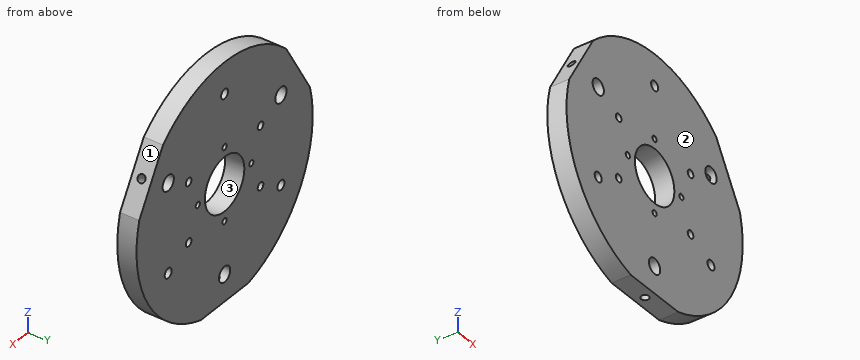
from build123d import *

# Parameters (mm, degrees)
SKETCH1_R           = 62.5
SKETCH1_R_2         = 4
BOSS_EXTRUDE1_DEPTH = 10
SKETCH2_W           = 43.972180284
SKETCH2_H           = 8.711954994
CUT_EXTRUDE1_DEPTH  = 10
SKETCH3_R           = 2
CUT_EXTRUDE2_DEPTH  = 12
SKETCH4_R           = 2
CUT_EXTRUDE3_DEPTH  = 12
SKETCH5_R           = 2
CUT_EXTRUDE4_DEPTH  = 12
SKETCH6_R           = 14
CUT_EXTRUDE5_DEPTH  = 12
SKETCH7_R           = 1.5
CUT_EXTRUDE6_DEPTH  = 10
SKETCH8_R           = 2
CUT_EXTRUDE7_DEPTH  = 10
SKETCH9_R           = 2.5
CUT_EXTRUDE8_DEPTH  = 10


with BuildPart() as part:
    # Sketch1 → Boss-Extrude1 (new body)
    with BuildSketch(Plane(origin=(0, 0, 0), x_dir=(1, 0, 0), z_dir=(0, 1, 0))):
        with Locations(Location((0, 0, 0), (0, 0, 270))):
            Circle(SKETCH1_R)
        with Locations(Location((0, 46.188021535, 0), (0, 0, 270))):
            Circle(SKETCH1_R_2, mode=Mode.SUBTRACT)
        with Locations(Location((40, -23.094010768, 0), (0, 0, 270))):
            Circle(SKETCH1_R_2, mode=Mode.SUBTRACT)
        with Locations(Location((-40, -23.094010768, 0), (0, 0, 270))):
            Circle(SKETCH1_R_2, mode=Mode.SUBTRACT)
    extrude(amount=BOSS_EXTRUDE1_DEPTH)

    # Sketch2 → Cut-Extrude1 (cut)
    with BuildSketch(Plane(origin=(0, 10, 0), x_dir=(1, 0, 0), z_dir=(0, 1, 0))):
        Polygon((-39.581845605, -51.818275424), (-64.713070734, -8.289716646), (-77.687460418, -15.780484023), (-52.55623529, -59.309042801), align=None)
        Polygon((40.609652539, -50.038061596), (63.321086643, -10.700703814), (75.641288558, -17.813775707), (52.929854454, -57.151133488), align=None)
        with Locations((0.471086747, 64.543999032)):
            Rectangle(SKETCH2_W, SKETCH2_H)
    extrude(amount=-CUT_EXTRUDE1_DEPTH, mode=Mode.SUBTRACT)

    # Sketch3 → Cut-Extrude2 (cut)
    with BuildSketch(Plane(origin=(52.124355653, 0, 30.094010768), x_dir=(0.49999999999999983, 0, -0.8660254037844387), z_dir=(0.8660254037844387, 0, 0.49999999999999983))):
        with Locations((0.001973272, 5)):
            Circle(SKETCH3_R)
    extrude(amount=-CUT_EXTRUDE2_DEPTH, mode=Mode.SUBTRACT)

    # Sketch4 → Cut-Extrude3 (cut)
    with BuildSketch(Plane(origin=(-52.124355653, 0, 30.094010768), x_dir=(0.5000000000000002, 0, 0.8660254037844386), z_dir=(-0.8660254037844385, 0, 0.5000000000000001))):
        with Locations((-0.001973272, 5)):
            Circle(SKETCH4_R)
    extrude(amount=-CUT_EXTRUDE3_DEPTH, mode=Mode.SUBTRACT)

    # Sketch5 → Cut-Extrude4 (cut)
    with BuildSketch(Plane(origin=(0, 0, -60.188021535), x_dir=(-1, 0, 0), z_dir=(0, 0, -1))):
        with Locations((-0.001973272, 5)):
            Circle(SKETCH5_R)
    extrude(amount=-CUT_EXTRUDE4_DEPTH, mode=Mode.SUBTRACT)

    # Sketch6 → Cut-Extrude5 (cut)
    with BuildSketch(Plane(origin=(0, 10, 0), x_dir=(1, 0, 0), z_dir=(0, 1, 0))):
        with Locations(Location((0, 0, 0), (0, 0, 270))):
            Circle(SKETCH6_R)
    extrude(amount=-CUT_EXTRUDE5_DEPTH, mode=Mode.SUBTRACT)

    # Sketch7 → Cut-Extrude6 (cut)
    with BuildSketch(Plane(origin=(0, 10, 0), x_dir=(1, 0, 0), z_dir=(0, 1, 0))):
        with Locations(Location((0, 19, 0), (0, 0, 270))):
            Circle(SKETCH7_R)
        with Locations(Location((19, 0, 0), (0, 0, 270))):
            Circle(SKETCH7_R)
        with Locations(Location((0, -19, 0), (0, 0, 270))):
            Circle(SKETCH7_R)
        with Locations(Location((-19, 0, 0), (0, 0, 270))):
            Circle(SKETCH7_R)
    extrude(amount=-CUT_EXTRUDE6_DEPTH, mode=Mode.SUBTRACT)

    # Sketch8 → Cut-Extrude7 (cut)
    with BuildSketch(Plane(origin=(0, 10, 0), x_dir=(1, 0, 0), z_dir=(0, 1, 0))):
        with Locations(Location((-25.5, 15.5, 0), (0, 0, 270))):
            Circle(SKETCH8_R)
        with Locations(Location((25.5, 15.5, 0), (0, 0, 270))):
            Circle(SKETCH8_R)
        with Locations(Location((25.5, -15.5, 0), (0, 0, 270))):
            Circle(SKETCH8_R)
        with Locations(Location((-25.5, -15.5, 0), (0, 0, 270))):
            Circle(SKETCH8_R)
    extrude(amount=-CUT_EXTRUDE7_DEPTH, mode=Mode.SUBTRACT)

    # Sketch9 → Cut-Extrude8 (cut)
    with BuildSketch(Plane(origin=(0, 10, 0), x_dir=(1, 0, 0), z_dir=(0, 1, 0))):
        with Locations(Location((-40, 23.094010768, 0), (0, 0, 270))):
            Circle(SKETCH9_R)
        with Locations(Location((40, 23.094010768, 0), (0, 0, 270))):
            Circle(SKETCH9_R)
        with Locations(Location((0, -46.188021535, 0), (0, 0, 270))):
            Circle(SKETCH9_R)
    extrude(amount=-CUT_EXTRUDE8_DEPTH, mode=Mode.SUBTRACT)


solid = part.part
Here's how the part is built. I have some questions about the finished solid (model axes, mm). Face numbers are marked on the shaded views. Coordinates: 2 decimals unless noted, no trailing zeros. Write each loop counter-clockwise with the first axis right and the second up, starting at its lowest first coordinate (ties: lowest second). Pieces come first, ordered by that corner, then holes.
1) Thinking about a two-plate mould opening in Z: for the marked faces 1, 2 and 3, which applies, +Z half, -Z half, draft (parallel to the pull), parting line (faces both ways), or undercut?
Filled in:
face 1: +Z half
face 2: draft
face 3: undercut
2) If we section it at A-A (x = 7): List the corners of the cut face in (y, z) for me, plus the area to 3 significant figures.
Filled in:
outline: (0, -60.19) - (10, -60.19) - (10, -12.12) - (0, -12.12) - close; (0, 12.12) - (10, 12.12) - (10, 62.11) - (0, 62.11) - close
area: 980 mm2
3) I'm going to push flat-ended pins straight in: pin 1 (6 mm diameter, centred on x = 47, y = 7.5, fed in from -Z); pin 2 (1 mm diameter, centred on x = 5.5, y = 4, fed in from +Z); pin 3 (6 mm diameter, centred on y = 3.5, z = 25.5, fed in from +X). Where does each tip first touch, or does it pass through?
Filled in:
pin 1: stops at z = -44.39
pin 2: stops at z = 62.3
pin 3: stops at x = 56.51
4) If we section it at B-B (z = 46.5): List the corners of the cut face in (x, y) for me.
Filled in:
outline: (-41.76, 0) - (-2.48, 0) - (-2.48, 10) - (-41.76, 10) - close; (2.48, 0) - (41.76, 0) - (41.76, 10) - (2.48, 10) - close
5) If I drill on line 1 (X direction, y = 2, z = 15.5); line 2 (X direction, y = 7.5, z = 0); line 3 (X direction, y = 2.25, z = 21), over which ranges is the centre line in solid material (lowest first)?
Filled in:
line 1: x = -60.55 to -27.5, -23.5 to 23.5, 27.5 to 60.55
line 2: x = -62.5 to -20.5, -17.5 to -14, 14 to 17.5, 20.5 to 62.5
line 3: x = -57.37 to -43.41, -36.59 to 36.59, 43.41 to 57.37
6) If we section it at D-D (z = -15.5): List the corners of the cut face in (x, y) for me.
Filled in:
outline: (-60.55, 0) - (-27.5, 0) - (-27.5, 10) - (-60.55, 10) - close; (-23.5, 0) - (23.5, 0) - (23.5, 10) - (-23.5, 10) - close; (27.5, 0) - (60.55, 0) - (60.55, 10) - (27.5, 10) - close
7) If we section it at C-C (x = -40): List the corners of the cut face in (y, z) for me.
Filled in:
outline: (0, -48.02) - (10, -48.02) - (10, -25.59) - (0, -25.59) - close; (0, -20.59) - (10, -20.59) - (10, 19.09) - (0, 19.09) - close; (0, 27.09) - (10, 27.09) - (10, 48.02) - (0, 48.02) - close
